from build123d import *

# Parameters (mm, degrees)
SKETCH1_R           = 96.15
BOSS_EXTRUDE1_DEPTH = 5
SKETCH2_R           = 88.15
CUT_EXTRUDE1_DEPTH  = 3
REVOLVE1_ANGLE      = 25
CIRPATTERN1_COUNT   = 3
FILLET1_R           = 10
SKETCH4_R           = 4
SKETCH4_R_2         = 1.4
BOSS_EXTRUDE2_DEPTH = 20
CHAMFER1_SIZE       = 1
BOSS_EXTRUDE3_DEPTH = 15
CUT_EXTRUDE2_DEPTH  = 15
CUT_EXTRUDE3_DEPTH  = 138.744854729
FILLET2_R           = 10
FILLET3_R           = 2
FILLET4_R           = 6
CUT_EXTRUDE4_DEPTH  = 15


with BuildPart() as part:
    # Sketch1 → Boss-Extrude1 (new body)
    with BuildSketch(Plane(origin=(0, 0, 0), x_dir=(1, 0, 0), z_dir=(0, 1, 0))):
        with Locations(Location((0, 0, 0), (0, 0, 270))):
            Circle(SKETCH1_R)
    extrude(amount=BOSS_EXTRUDE1_DEPTH)

    # Sketch2 → Cut-Extrude1 (cut)
    with BuildSketch(Plane(origin=(0, 5, 0), x_dir=(1, 0, 0), z_dir=(0, 1, 0))):
        with Locations(Location((0, 0, 0), (0, 0, 270))):
            Circle(SKETCH2_R)
    extrude(amount=-CUT_EXTRUDE1_DEPTH, mode=Mode.SUBTRACT)

    # Sketch3 → Revolve1 (revolve)
    with BuildSketch(Plane.XY):
        Polygon((-88.15, 2), (-88.15, 15), (-88.877940469, 17), (-88.877940469, 22), (-88.15, 24), (-86.15, 24), (-85.15, 2), align=None)
    revolve1 = revolve(axis=Axis((0, 2, 0), (0, 1, 0)), revolution_arc=REVOLVE1_ANGLE)

    # CirPattern1: Revolve1 ×3 about axis
    cirpattern1_axis = Axis((0, 0, 0), (0, 1, 0))
    for i in range(1, CIRPATTERN1_COUNT):
        add(revolve1.rotate(cirpattern1_axis, i * 360 / CIRPATTERN1_COUNT))

    # Fillet1
    fillet1_edges = [part.edges().sort_by_distance(p)[0] for p in [
        (-83.131605006, 2, 18.429833127),
        (57.526506178, 2, 62.779165229),
        (25.605098828, 2, -81.208998356),
    ]]
    fillet(fillet1_edges, radius=FILLET1_R)

    # Sketch4 → Boss-Extrude2 (add)
    # profile 1 of 4: a face of its own
    with BuildSketch(Plane(origin=(0, 2, 0), x_dir=(1, 0, 0), z_dir=(0, 1, 0))):
        with Locations(Location((-36.838329564, 24.647548103, 0), (0, 0, 270))):
            Circle(SKETCH4_R)
        with Locations(Location((-36.838329564, 24.647548103, 0), (0, 0, 270))):
            Circle(SKETCH4_R_2, mode=Mode.SUBTRACT)
    # profile 2 of 4: a face of its own
    with BuildSketch(Plane(origin=(0, 2, 0), x_dir=(1, 0, 0), z_dir=(0, 1, 0))):
        with Locations(Location((44.313445776, -0.939508377, 0), (0, 0, 270))):
            Circle(SKETCH4_R)
        with Locations(Location((44.313445776, -0.939508377, 0), (0, 0, 270))):
            Circle(SKETCH4_R_2, mode=Mode.SUBTRACT)
    # profile 3 of 4: a face of its own
    with BuildSketch(Plane(origin=(0, 2, 0), x_dir=(1, 0, 0), z_dir=(0, 1, 0))):
        with Locations(Location((25.218627507, -61.50053475, 0), (0, 0, 270))):
            Circle(SKETCH4_R)
        with Locations(Location((25.218627507, -61.50053475, 0), (0, 0, 270))):
            Circle(SKETCH4_R_2, mode=Mode.SUBTRACT)
    # profile 4 of 4: a face of its own
    with BuildSketch(Plane(origin=(0, 2, 0), x_dir=(1, 0, 0), z_dir=(0, 1, 0))):
        with Locations(Location((-55.933147832, -35.91347827, 0), (0, 0, 270))):
            Circle(SKETCH4_R)
        with Locations(Location((-55.933147832, -35.91347827, 0), (0, 0, 270))):
            Circle(SKETCH4_R_2, mode=Mode.SUBTRACT)
    extrude(amount=BOSS_EXTRUDE2_DEPTH)

    # Chamfer1
    chamfer1_edges = [part.edges().sort_by_distance(p)[0] for p in [
        (0, 0, -96.15),
    ]]
    chamfer(chamfer1_edges, length=CHAMFER1_SIZE)

    # Sketch5 → Boss-Extrude3 (add)
    with BuildSketch(Plane(origin=(0, 2, 0), x_dir=(1, 0, 0), z_dir=(0, 1, 0))):
        Polygon((9.002514728, -81.887842353), (42.723663084, 25.061976503), (-20.622216784, 45.034855706), (-54.343365141, -61.91496315), align=None)
        Polygon((6.390470123, -76.870151352), (-49.32567414, -59.302918545), (-18.010172179, 40.017164705), (37.705972083, 22.449931898), align=None, mode=Mode.SUBTRACT)
    extrude(amount=BOSS_EXTRUDE3_DEPTH)

    # Sketch6 → Cut-Extrude2 (cut)
    with BuildSketch(Plane(origin=(0, 17, 0), x_dir=(1, 0, 0), z_dir=(0, 1, 0))):
        Polygon((28.721958407, 25.28258053), (29.924781605, 29.097448333), (-8.223896425, 41.125680313), (-9.426719623, 37.31081251), align=None)
        Polygon((34.698914088, 12.912762391), (37.705972083, 22.449931898), (41.520839886, 21.2471087), (38.513781891, 11.709939193), align=None)
    extrude(amount=-CUT_EXTRUDE2_DEPTH, mode=Mode.SUBTRACT)

    # Sketch7 → Cut-Extrude3 (cut, through all)
    with BuildSketch(Plane(origin=(0, 2, 0), x_dir=(1, 0, 0), z_dir=(0, 1, 0))):
        Polygon((39.287775175, -35.717910583), (57.029417346, 20.551389511), (85.640925868, 11.530215526), (67.899283697, -44.739084568), align=None)
    extrude(amount=-CUT_EXTRUDE3_DEPTH, mode=Mode.SUBTRACT)

    # Fillet2
    fillet2_edges = [part.edges().sort_by_distance(p)[0] for p in [
        (67.899283697, 1, 44.739084568),
        (39.287775175, 1, 35.717910583),
        (57.029417346, 1, -20.551389511),
        (85.640925868, 1, -11.530215526),
    ]]
    fillet(fillet2_edges, radius=FILLET2_R)

    # Fillet3
    fillet3_edges = [part.edges().sort_by_distance(p)[0] for p in [
        (-36.838329564, 2, -28.647548103),
        (44.313445776, 2, -3.060491623),
        (25.218627507, 2, 57.50053475),
        (-55.933147832, 2, 31.91347827),
    ]]
    fillet(fillet3_edges, radius=FILLET3_R)

    # Fillet4
    fillet4_edges = [part.edges().sort_by_distance(p)[0] for p in [
        (20.544692106, 2, 31.978694481),
        (-33.66792316, 2, 9.64287692),
    ]]
    fillet(fillet4_edges, radius=FILLET4_R)

    # Sketch8 → Cut-Extrude4 (cut)
    with BuildSketch(Plane(origin=(0, 17, 0), x_dir=(1, 0, 0), z_dir=(0, 1, 0))):
        Polygon((-10.071824287, -75.873726363), (-35.269026126, -67.92907914), (-34.066202928, -64.114211338), (-8.869001089, -72.05885856), align=None)
    extrude(amount=-CUT_EXTRUDE4_DEPTH, mode=Mode.SUBTRACT)


solid = part.part
CAD build for the part. Positions are in the model's coordinates, mm. A direction names the side the tool comes from. Coordinates: 2 decimals unless noted, no trailing zeros.
Item 1: 3-axis set-ups, long thin cutter, end or side, ignore diameter. For faces 1 (the face through (59.549, 15.792, 65.386)), 2 (the face through (-86.83, 19.54, 18.97)), 3 (the face through (20.743, 12.437, 31.35)): which of +Z, -Z, +X, -X, +Y, -Y reach the whole face in a straight line?
Check sheet entries:
face 1: +Z, +X
face 2: +Z, -X, +Y
face 3: +Y
Item 2: Drill centre lines: L1, parallel to X at y = 14, z = 19; L2, parallel to X at y = 15, z = 16; L3, parallel to X at y = 2.5, z = -11. Where is each one in solid material? Low to high.
Check sheet entries:
L1: x = -86.08 to -83.56, -40.81 to -36.62, 24.64 to 28.83
L2: x = -86.69 to -84.23, -39.87 to -35.67, 25.58 to 29.78
L3: x = -95.52 to -87.46, -31.35 to -23.38, 30.32 to 38.29, 87.46 to 95.52
Item 3: Two-plate mould, pull along Y, no slides. Class faces 4 (the face through (-86.118, 10.07, 18.816)), 5 (the face through (1, 2, -1)), 6 (the face through (-59.48, 12.87, 37.76)): +Y half, -Y half, draft (parallel to the pull), parting line (faces both ways), or undercut.
Check sheet entries:
face 4: undercut
face 5: +Y half
face 6: draft
Item 4: Pin check, flat tips, straight feed: pin 1 Ø1.5 at (y, z) = (7.5, -9) entering from -X; pin 2 Ø2 at (x, z) = (25.22, 61.5) entering from +Y; pin 3 Ø10 at (x, y) = (11.5, 12.5) entering from -Z; pin 4 Ø1.5 at (x, z) = (-12, 71.5) entering from -Y. Stop position of each tip, or through.
Check sheet entries:
pin 1: stops at x = -32.22
pin 2: stops at y = 2
pin 3: stops at z = -88.39
pin 4: stops at y = 0
